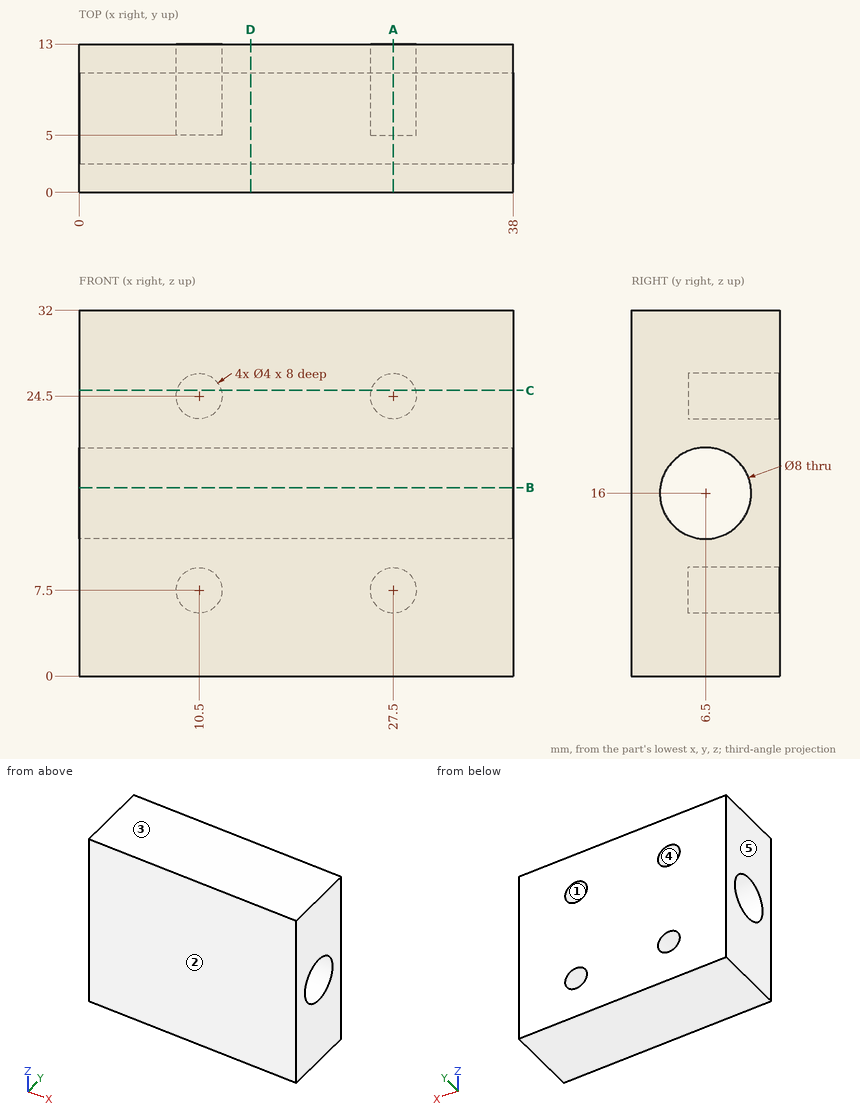
Check sheet for the drawn part. Datum: minimum x, y, z corner. Units: mm. A direction names the side the tool comes from. Coordinates: 2 decimals unless noted, no trailing zeros. Loops run counter-clockwise (first coordinate to the right, second up) from the corner with the lowest first, then second, coordinate; pieces in that order, holes last. Notation, with made-up numbers: (52.25, 82) -> (70.25, 82) arc R21 cw to (70.25, 111) -> close; hole circle Ø5 at (13.25, 86.5). An arc over 180 degrees is marked (long way). Answer as a JSON object with one key per item and string values. Group by question number.
Item 1: Depth check by flat-ended pin: pin 1 (7 mm diameter, centred on y = 6.5, z = 16, fed in from +X); pin 2 (1.2 mm diameter, centred on x = 27.5, z = 25, fed in from +Y). Enter the tip coordinate at first touch or a pass-through.
Item 2: Scan lines: probe 1 along X at (y, z) = (10.75, 7.5); probe 2 along Z at (x, y) = (27, 8); probe 3 along Y at (x, z) = (23, 16). Record each from-to range of solid material in increasing order.
Item 3: Sectioned sample at C-C on z = 25. Record the boundary of the cut face in (x, y), plus the area to 3 significant figures.
Item 4: Sectioned sample at B-B on z = 16.5. Record the boundary of the cut face in (x, y).
Item 5: Mould release check, pull along X, two halves, no side actions. Record for the marked faces 3, 4 and 5: +X half, -X half, draft (parallel to the pull), parting line (faces both ways), or undercut.
Item 6: Tool access check on the marked faces 1 and 2. Record the directions out of +Z, -Z, +X, -X, +Y, -Y that give a thin tool (end or side, any length) a straight path to the whole face; none if there is none.
Item 7: Sectioned sample at D-D on x = 15. Record the boundary of the cut face in (y, z).
Item 8: Sectioned sample at A-A on x = 27.5. Record the boundary of the cut face in (y, z).
Evaluation:
{
 "1": {"pin 1": "passes through", "pin 2": "stops at y = 5"},
 "2": {"probe 1": "x = 0 to 8.5, 12.5 to 25.5, 29.5 to 38", "probe 2": "z = 0 to 5.56, 9.44 to 12.29, 19.71 to 22.56, 26.44 to 32", "probe 3": "y = 0 to 2.5, 10.5 to 13"},
 "3": {"outline": "(0, 0) -> (38, 0) -> (38, 13) -> (29.44, 13) -> (29.44, 5) -> (25.56, 5) -> (25.56, 13) -> (12.44, 13) -> (12.44, 5) -> (8.56, 5) -> (8.56, 13) -> (0, 13) -> close", "area": "432 mm²"},
 "4": {"outline": "(0, 0) -> (38, 0) -> (38, 2.53) -> (0, 2.53) -> close; (0, 10.47) -> (38, 10.47) -> (38, 13) -> (0, 13) -> close"},
 "5": {"face 3": "draft", "face 4": "undercut", "face 5": "-X half"},
 "6": {"face 1": "+Y", "face 2": "+Z, -Z, +X, -X, -Y"},
 "7": {"outline": "(0, 0) -> (13, 0) -> (13, 32) -> (0, 32) -> close; hole circle Ø8 at (6.5, 16)"},
 "8": {"outline": "(0, 0) -> (13, 0) -> (13, 5.5) -> (5, 5.5) -> (5, 9.5) -> (13, 9.5) -> (13, 22.5) -> (5, 22.5) -> (5, 26.5) -> (13, 26.5) -> (13, 32) -> (0, 32) -> close; hole circle Ø8 at (6.5, 16)"}
}
